Read the model definition and answer for the solid it produces. Units are mm, in the model's axes. A direction names the side the tool comes from. Coordinates: 2 decimals unless noted, no trailing zeros. Loops run counter-clockwise (first coordinate to the right, second up) from the corner with the lowest first, then second, coordinate; pieces in that order, holes last. Notation, with made-up numbers: (38, 12) -> (91, 12) arc R25 cw to (91, 49) -> close; hole circle Ø5 at (25.5, -17). An arc over 180 degrees is marked (long way). Answer as CSV lines item,"result".
Solid Edge part; units mm, degrees
sketch "Sketch1" plane through (0, 0, 0) normal (0, -1, 0) x (1, 0, 0)
  line L0 (140, -140) -> (140, 140)
  line L1 (140, 140) -> (-140, 140)
  line L2 (-140, 140) -> (-140, -140)
  line L3 (-140, -140) -> (140, -140)
  line L4 (150, -150) -> (150, 150)
  line L5 (150, 150) -> (-150, 150)
  line L6 (-150, 150) -> (-150, -150)
  line L7 (-150, -150) -> (150, -150)
extrude "Protrusion1" add sketch "Sketch1" along normal blind 300
sketch "Sketch2" plane through (0, -150, 150) normal (0, 0, 1) x (1, 0, 0)
  line L0 (7.5, -125) -> (7.5, 125)
  line L1 (7.5, 125) -> (-7.5, 125)
  line L2 (-7.5, 125) -> (-7.5, -125)
  line L3 (-7.5, -125) -> (7.5, -125)
extrude "Cutout1" cut sketch "Sketch2" against normal up to next
Q1. A cutting plane is placed at A-A, the plane x = -78. Write down the section's boundary in (y, z).
Results:
outline,"(-300, -150) -> (0, -150) -> (0, -140) -> (-300, -140) -> close; (-300, 140) -> (0, 140) -> (0, 150) -> (-300, 150) -> close"
Q2. For faces 5 (the face through (0, -275, 145)), 6 (the face through (-29, -148, 140)), 7 (the face through (-144, -300, 12)), determine the directions among +Z, -Z, +X, -X, +Y, -Y from which every point of the face is accessible in a straight line to the end or side of a thin tool.
Results:
face 5,"+Z"
face 6,"+Y, -Y"
face 7,"+Z, -Z, +X, -X, -Y"
Q3. A cutting plane is placed at C-C, the plane z = 101. Write down the section's boundary in (x, y), and give its area (3 significant figures).
Results:
outline,"(-150, -300) -> (-140, -300) -> (-140, 0) -> (-150, 0) -> close; (140, -300) -> (150, -300) -> (150, 0) -> (140, 0) -> close"
area,"6,000 mm²"
Q4. A cutting plane is placed at D-D, the plane y = -84.5. Write down the section's boundary in (x, z), and give its area (4 significant figures).
Results:
outline,"(-150, -150) -> (150, -150) -> (150, 150) -> (7.5, 150) -> (7.5, 140) -> (140, 140) -> (140, -140) -> (-140, -140) -> (-140, 140) -> (-7.5, 140) -> (-7.5, 150) -> (-150, 150) -> close"
area,"11,450 mm²"
Q5. A cutting plane is placed at B-B, the plane y = -19. Write down the section's boundary in (x, z), and give its area (3 significant figures).
Results:
outline,"(-150, -150) -> (150, -150) -> (150, 150) -> (-150, 150) -> close; hole (-140, -140) -> (140, -140) -> (140, 140) -> (-140, 140) -> close"
area,"11,600 mm²"
Q6. For a pull along Z with two mould halves and no side action, classify faces 1 (the face through (-140, -148, 2)), 2 (the face through (-7.5, -148, 145)), 3 (the face through (-2, -148, -150)), 4 (the face through (140, -148, -2)) as pulls with the +Z half, pulls with the -Z half, needs draft (parallel to the pull), parting line crosses it, or undercut.
Results:
face 1,"undercut"
face 2,"needs draft"
face 3,"pulls with the -Z half"
face 4,"undercut"
Q7. Find the intervals of material crossed by probe 1 along Z at (x, y) = (118, -64.5); probe 2 along Z at (x, y) = (-5, -96.5), in increasing order. Write a range as [from, to].
Results:
probe 1,"z = [-150, -140], [140, 150]"
probe 2,"z = [-150, -140]"
